Autodesk Inventor part; units mm, degrees
ref_plane "YZ Plane" through (0, 0, 0) normal (1, 0, 0) x (0, 1, 0)
ref_plane "XZ Plane" through (0, 0, 0) normal (0, 1, 0) x (-1, 0, 0)
ref_plane "XY Plane" through (0, 0, 0) normal (0, 0, 1) x (1, 0, 0)
sketch "Sketch1" plane through (0, 0, 0) normal (0, 1, 0) x (-1, 0, 0)
  line L0 (-4.1, 0) -> (-35.9, 0)
  line L1 (-40, -4.1) -> (-40, -4.1)
  line L2 (-35.9, -8.2) -> (-4.1, -8.2)
  line L3 (0, -4.1) -> (0, -4.1)
  circle A0 centre (-35.9, -4.1) radius 2.05
  circle A1 centre (-4.1, -4.1) radius 1.75
  arc A2 (-4.1, -8.2) -> (0, -4.1) centre (-4.1, -4.1) ccw
  arc A3 (0, -4.1) -> (-4.1, 0) centre (-4.1, -4.1) ccw
  arc A4 (-35.9, 0) -> (-40, -4.1) centre (-35.9, -4.1) ccw
  arc A5 (-40, -4.1) -> (-35.9, -8.2) centre (-35.9, -4.1) ccw
  point P0 (0, 0)
  point P1 (-40, -8.2)
  point P2 (-40, 0)
  point P3 (0, -8.2)
  point P4 (-40, -4.1)
  point P5 (0, -4.1)
  dimension "d0" = 40
  dimension "d1" = 8.2
  dimension "d2" = 4.1
  dimension "d3" = 3.5
  dimension "d4" = 4.1
  dimension "d5" = 4.1
  dimension "d6" = 4.1
  dimension "d7" = 4.1
  dimension "d8" = 4.1
extrude "Extrusion1" add sketch "Sketch1" along normal blind 4
equation "\"d2\" = arm_rod_diam"
equation "\"d4\" = 0.5 * d1"
equation "\"d5\" = d4"
equation "\"d6\" = d4"
equation "\"d7\" = d5"
equation "\"d8\" = arm_rod_diam"
equation "\"arm_rod_diam\" = 4.1"
properties part number "config_arm" material "ABS Plastic"
For this review, take the finished solid that the model builds, in its own axes (mm). Give positions to 0.01 mm unless a question says otherwise; leave off trailing zeros. Loops run counter-clockwise (first coordinate to the right, second up) from the corner with the lowest first, then second, coordinate; pieces in that order, holes last.
Item 1: Insertion check: pin 1 (1 mm diameter, centred on y = 2, z = -3, fed in from +X); pin 2 (1.5 mm diameter, centred on y = 2.5, z = -2.5, fed in from -X). Each pin has a flat end and moves straight along its axis. Give the tip position at first contact, or say it passes through.
Item 2: Take a section at B-B, the plane y = 0.5. State the section outline as (x, z) points, and give its area (3 significant figures).
Item 3: Take a section at C-C, the plane x = 37.5. State the section outline as (y, z) points.
Item 4: Take a section at A-A, the plane z = -4.1. State the section outline as (x, y) points, and give its area (3 significant figures).
Item 5: Take a section at D-D, the plane z = -6.5. State the section outline as (x, y) points.
Item 6: For line 1 along X through (y, z) = (1.45, -4.75); line 2 along Z through (x, y) = (35.9, 2.85); line 3 along X through (y, z) = (3.05, -3.75), list the stretches that pass through material, from the lowest coordinate up.
Item 7: Draft analysis for pull direction Z (two halves, no side actions). For faces 1 (the flat face through (20, 4, -4)), 2 (the cylindrical face through (3.2, 2, -5.6)), 3 (the flat face through (20, 2, 0)), state which applies: +Z half, -Z half, draft (parallel to the pull), parting line (faces both ways), or undercut.
Calculated:
1. pin 1: stops at x = 39.96
1. pin 2: stops at x = 0.09
2. outline: (4.1, -8.2) - (35.9, -8.2) arc R4.1 ccw to (35.9, 0) - (4.1, 0) arc R4.1 ccw to start; hole circle Ø3.5 at (4.1, -4.1); hole circle Ø4.1 at (35.9, -4.1)
2. area: 291 mm2
3. outline: (0, -7.87) - (4, -7.87) - (4, -5.38) - (0, -5.38) - close; (0, -2.82) - (4, -2.82) - (4, -0.33) - (0, -0.33) - close
4. outline: (0, 0) - (2.35, 0) - (2.35, 4) - (0, 4) - close; (5.85, 0) - (33.85, 0) - (33.85, 4) - (5.85, 4) - close; (37.95, 0) - (40, 0) - (40, 4) - (37.95, 4) - close
4. area: 130 mm2
5. outline: (0.78, 0) - (39.22, 0) - (39.22, 4) - (0.78, 4) - close
6. line 1: x = 0.05 to 2.48, 5.72 to 33.96, 37.84 to 39.95
6. line 2: z = -8.2 to -6.15, -2.05 to 0
6. line 3: x = 0.01 to 2.39, 5.81 to 33.88, 37.92 to 39.99
7. face 1: draft
7. face 2: undercut
7. face 3: +Z half
